```python
from build123d import *

# Parameters (mm, degrees)
F0_W     = 600
F0_H     = 300
F1_DEPTH = 10
F2_W     = 600
F2_H     = 10
F2_H_2   = 20
F3_DEPTH = 10


with BuildPart() as f1:
    # F0 (on Top) → F1 (new body)
    with BuildSketch(Plane.XY):
        Rectangle(F0_W, F0_H)
    extrude(amount=F1_DEPTH)

    # F2 (on face) → F3 (join)
    with BuildSketch(Plane.XY):
        with Locations((0, -145)):
            Rectangle(F2_W, F2_H)
        with Locations((0, -155)):
            Rectangle(F2_W, F2_H)
        with Locations((0, 130)):
            Rectangle(F2_W, F2_H_2)
    extrude(amount=-F3_DEPTH)


solid = f1.part
```
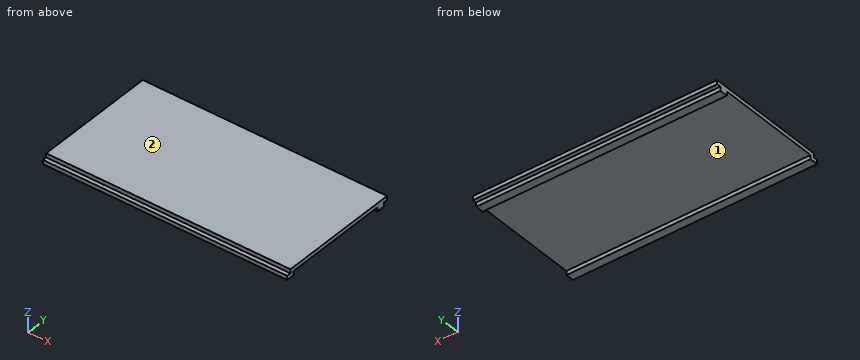
The listing builds one solid part. Answer for the finished solid, in the listing's coordinates (mm). Face numbers are marked on the shaded views. Give positions to 0.01 mm unless a question says otherwise; leave off trailing zeros. Write each loop counter-clockwise with the first axis right and the second up, starting at its lowest first coordinate (ties: lowest second). Pieces come first, ordered by that corner, then holes. Notation, with made-up numbers: (14.25, 55) - (34.25, 55) arc R13 ccw to (34.25, 76) - close; hole circle Ø2 at (-32, -39). An arc over 180 degrees is marked (long way). Use one line per item in the form item = value. Start each with the question number.
1) Find section A-A on z = -5.5. Determine the outline of the cut face in (x, y), plus the area to 3 significant figures.
2) Find section C-C on y = -8. Determine the outline of the cut face in (x, z).
3) Flat-ended cylindrical pins translate along their axes: pin 1 Ø5 at (x, z) = (-138, -3.5) entering from +Y; pin 2 Ø11 at (x, y) = (85.5, 147.5) entering from -Z; pin 3 Ø3 at (x, y) = (57, -154.5) entering from +Z. Find the tip coordinate at first contact, or state that the pin passes through.
4) Find section B-B on x = 10.5. Determine the outline of the cut face in (y, z).
5) The mould has two halves that part along Y. Classify the marked faces 1 and 2: pulls with the +Y half, pulls with the -Y half, needs draft (parallel to the pull), parting line crosses it, or undercut.
6) Consider line 1 along Y through (x, z) = (208, -1.25); line 2 along Y through (x, z) = (-16.5, 7.75); line 3 along Z through (x, y) = (-106, 92.5). Determine where each line is inside the solid, lowest interval first. Write a range as from..to.
Geometry results:
q1.outline = (-300, -160) - (300, -160) - (300, -140) - (-300, -140) - close; (-300, 120) - (300, 120) - (300, 140) - (-300, 140) - close
q1.area = 24,000 mm2
q2.outline = (-300, 0) - (300, 0) - (300, 10) - (-300, 10) - close
q3.pin_1 = 140
q3.pin_2 = 0
q3.pin_3 = 0
q4.outline = (-160, -10) - (-140, -10) - (-140, 0) - (120, 0) - (120, -10) - (140, -10) - (140, 0) - (150, 0) - (150, 10) - (-150, 10) - (-150, 0) - (-160, 0) - close
q5.face_1 = undercut
q5.face_2 = needs draft
q6.line_1 = -160..-140, 120..140
q6.line_2 = -150..150
q6.line_3 = 0..10
